Here's how the part is built. I have some questions about the finished solid (model axes, mm). Face numbers are marked on the shaded views. Coordinates: 2 decimals unless noted, no trailing zeros. Write each loop counter-clockwise with the first axis right and the second up, starting at its lowest first coordinate (ties: lowest second). Pieces come first, ordered by that corner, then holes. Notation, with made-up numbers: (56.25, -27) -> (107.25, -27) arc R29 ccw to (107.25, -3) -> close; hole circle Ø3 at (30, 3.25). An arc over 180 degrees is marked (long way). Use a Markdown table: item, result. Add a question column.
Item 1: Imagine slicing it at B-B, the plane x = 4. Write out the boundary of the cut face in (y, z), and give its area (3 significant figures).
Item 2: Imagine slicing it at D-D, the plane x = 6. Write out the boundary of the cut face in (y, z), and give its area (3 significant figures).
Item 3: If I drill on line 1 along Z through (x, y) = (6.5, -1.5); line 2 along Y through (x, z) = (4, -2.25); line 3 along Y through (x, z) = (5.25, -2.25), over which ranges is the centre line in solid material (lowest first)? Write a range as from..to.
Item 4: Imagine slicing it at A-A, the plane x = 1.5. Write out the boundary of the cut face in (y, z).
Item 5: Imagine slicing it at C-C, the plane x = 5. Write out the boundary of the cut face in (y, z), and give its area (3 significant figures).
Item 6: If we mould it in two halves opening along Z, with no side actions, what happens to the marked faces 1, 2, 3 and 4? For each: pulls with the +Z half, pulls with the -Z half, needs draft (parallel to the pull), parting line crosses it, or undercut.
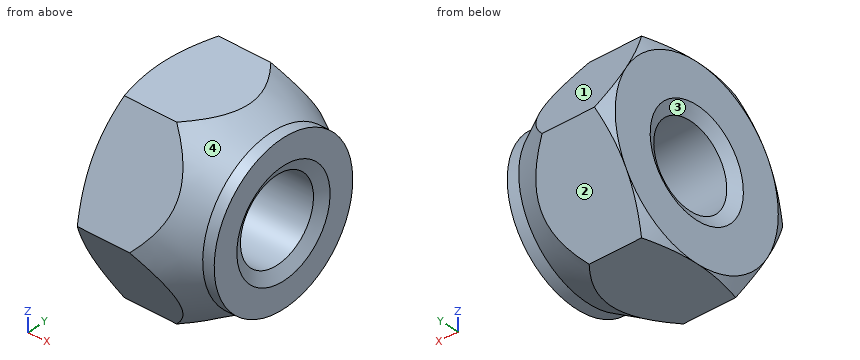
```python
from build123d import *

# Parameters (mm, degrees)
BODY_DEPTH     = 7.3152
THREAD_D       = 4.9784
CHAMFER1_SIZE  = 0.687407664
CHAMFER1_SIZE2 = 0.396875
CHAMFER2_SIZE  = 0.687407664
CHAMFER2_SIZE2 = 0.396875


with BuildPart() as part:
    # Sketch1 → Body (new body)
    with BuildSketch(Plane.YZ):
        Polygon((-6.415804866, 0), (-3.207902433, 5.55625), (3.207902433, 5.55625), (6.415804866, 0), (3.207902433, -5.55625), (-3.207902433, -5.55625), align=None)
    extrude(amount=BODY_DEPTH)

    # Thread (through all)
    with Locations(Plane.ZY):
        with Locations((0, 0)):
            Hole(THREAD_D / 2)

    # Chamfer1
    chamfer1_edges = [part.edges().sort_by_distance(p)[0] for p in [
        (0, 0, 2.4892),
    ]]
    chamfer1_side = [part.faces().sort_by_distance(p)[0] for p in [
        (0, -4.664849093, 2.693251879),
    ]]
    chamfer(chamfer1_edges, length=CHAMFER1_SIZE, length2=CHAMFER1_SIZE2, reference=chamfer1_side[0])

    # Chamfer2
    chamfer2_edges = [part.edges().sort_by_distance(p)[0] for p in [
        (7.3152, 0, 2.4892),
    ]]
    chamfer2_side = [part.faces().sort_by_distance(p)[0] for p in [
        (7.3152, -4.664849093, 2.693251879),
    ]]
    chamfer(chamfer2_edges, length=CHAMFER2_SIZE, length2=CHAMFER2_SIZE2, reference=chamfer2_side[0])

    # Sketch4 → Chamfer3 (revolve, cut)
    with BuildSketch(Plane.XY, mode=Mode.PRIVATE) as chamfer3_sk:
        Polygon((0, 5.55625), (0.496264233, 6.415804866), (0, 6.415804866), align=None)
        Polygon((7.3152, 4.7228125), (7.3152, 6.415804866), (3.683, 6.415804866), (6.615348795, 4.7228125), align=None)
    revolve(chamfer3_sk.sketch.rotate(Axis((-1.46304, 0, 0), (1, 0, 0)), 90), axis=Axis((-1.46304, 0, 0), (1, 0, 0)), mode=Mode.SUBTRACT)


solid = part.part
```
Ans:
| question | item | result |
|---|---|---|
| 1 | outline | (-6.22, -0.33) -> (-3.4, -5.22) arc R6.23 ccw to (-2.82, -5.56) -> (2.82, -5.56) arc R6.23 ccw to (3.4, -5.22) -> (6.22, -0.33) arc R6.23 ccw to (6.22, 0.33) -> (3.4, 5.22) arc R6.23 ccw to (2.82, 5.56) -> (-2.82, 5.56) arc R6.23 ccw to (-3.4, 5.22) -> (-6.22, 0.33) arc R6.23 ccw to start; hole circle Ø4.98 at (0, 0) |
| 1 | area | 87.1 mm^2 |
| 2 | outline | circle Ø10.16 at (0, 0); hole circle Ø4.98 at (0, 0) |
| 2 | area | 61.5 mm^2 |
| 3 | line 1 | z = -4.55..-1.99, 1.99..4.55 |
| 3 | line 2 | y = -5.12..-1.06, 1.06..5.12 |
| 3 | line 3 | y = -5.03..-1.06, 1.06..5.03 |
| 4 | outline | (-6.42, 0) -> (-3.21, -5.56) -> (3.21, -5.56) -> (6.42, 0) -> (3.21, 5.56) -> (-3.21, 5.56) -> close; hole circle Ø4.98 at (0, 0) |
| 5 | outline | (-5.34, -1.86) -> (-4.28, -3.69) arc R5.66 ccw to (-1.05, -5.56) -> (1.05, -5.56) arc R5.66 ccw to (4.28, -3.69) -> (5.34, -1.86) arc R5.66 ccw to (5.34, 1.86) -> (4.28, 3.69) arc R5.66 ccw to (1.05, 5.56) -> (-1.05, 5.56) arc R5.66 ccw to (-4.28, 3.69) -> (-5.34, 1.86) arc R5.66 ccw to start; hole circle Ø4.98 at (0, 0) |
| 5 | area | 80.2 mm^2 |
| 6 | face 1 | pulls with the +Z half |
| 6 | face 2 | pulls with the -Z half |
| 6 | face 3 | undercut |
| 6 | face 4 | parting line crosses it |
